Autodesk Fusion 360 part; units mm, degrees
sketch "Bottom back base" plane through (0, 0, 0) normal (0, 0, 1) x (1, 0, 0)
  line L0 (-60, 60) -> (-60, -60)
  line L1 (60, -20) -> (60, 20)
  line L2 (-60, 0) -> (-57.5, 0) construction
  line L3 (-57.5, -60) -> (-57.5, -6) construction
  line L4 (-57.5, -6) -> (12.5, -6) construction
  line L5 (12.5, -6) -> (12.5, -34) construction
  line L6 (12.5, -34) -> (30, -34)
  line L7 (30, -34) -> (12.5, -34)
  line L8 (12.5, -34) -> (-40, -34)
  line L9 (-40, -34) -> (-40, -60)
  line L10 (30, -34) -> (30, -60)
  line L11 (-40, 34) -> (-40, 60)
  line L12 (12.5, 34) -> (-40, 34)
  line L13 (12.5, 34) -> (30, 34)
  line L14 (30, 34) -> (30, 60)
  line L15 (50, -60) -> (60, -20)
  line L16 (50, 60) -> (60, 20)
  line L17 (50, 60) -> (30, 60)
  line L18 (-40, 60) -> (-60, 60)
  line L19 (-60, -60) -> (-40, -60)
  line L20 (30, -60) -> (50, -60)
  point P0 (60, 60)
  point P1 (60, -60)
  dimension "d1" = 120
  dimension "d2" = 120
  dimension "d3" = 2.5
  dimension "d4" = 54
  dimension "d5" = 70
  dimension "d6" = 28
  dimension "d8" = 70
  dimension "d9" = 10
  dimension "d10" = 40
  dimension "d11" = 10
  dimension "d12" = 40
extrude "Bottom back height" add sketch "Bottom back base" along normal blind 5
sketch "Connector" plane through (-60, 0, 0) normal (-1, 0, 0) x (0, -1, 0)
  line L0 (-60, 0) -> (60, 0)
  line L1 (60, 0) -> (60, 5)
  line L2 (60, 5) -> (-60, 5)
  line L3 (-60, 5) -> (-60, 0)
  line L4 (0, 0) -> (0, 5) construction
  line L5 (30, 4) -> (-30, 4)
  line L6 (-30, 4) -> (-30, 1)
  line L7 (-30, 1) -> (30, 1)
  line L8 (30, 1) -> (30, 4)
  line L9 (30, 4) -> (-30, 1) construction
  line L10 (-30, 4) -> (30, 1) construction
  point P0 (0, 2.5)
  dimension "d15" = 3
  dimension "d16" = 60
extrude "Connector width" add sketch "Connector" along normal blind 60 contours L5 L6 L7 L8
equation "d6 = 54 mm - 26 mm"
Geometry: final body of the model. Coordinates: model frame, mm. A direction names the side the tool comes from. Round coordinates to 2 decimals unless told otherwise and drop trailing zeros. Order: outer loops, then holes, each group sorted by start corner. A loop starts at its lowest first (then second) coordinate and runs counter-clockwise, first axis right, second up. Notation, with made-up numbers: M 23.25,-6.5 L 47.25,-6.5 A31 cw 47.25,17.5 Z; hole C 42,64 d3. An arc over 180 degrees is marked long. Use one line per item in the form item = value. Start each with the question number.
Q1. Pin query (flat end, axial travel): pin 1 Ø2.5 at (y, z) = (42.5, 3.5) entering from +X; pin 2 Ø2 at (x, z) = (-96.5, 1.5) entering from -Y; pin 3 Ø2.5 at (y, z) = (-49, 3.5) entering from +X. Return the tip coordinate at first contact, or that it passes through.
Q2. Cut plane D-D (x = -8). Return loops of the section in (y, z), and give its area (3 significant figures).
Q3. Mould query, pull axis X, two halves, no side actions, for faces 1 (the face through (-40, 47, 2)), 2 (the face through (-5, 34, 2)), 3 (the face through (60, 0, 2)), 4 (the face through (-90, 0, 4)). Classes: +X half, -X half, draft (parallel to the pull), parting line (faces both ways), or undercut.
Q4. Cut plane B-B (y = -10). Return loops of the section in (x, z), and give its area (3 significant figures).
Q5. Cut plane C-C (z = 2). Return loops of the section in (x, y).
Q6. Access query for faces 5 (the face through (-90, 0, 1)), 6 (the face through (-40, -47, 2)), 7 (the face through (30, 47, 2)). Directions: +Z, -Z, +X, -X, +Y, -Y. A direction counts if a zero-diameter tool reaches every point of the face in a straight line with its end or side. Return the directions, or none.
Q7. Cut plane A-A (y = -38.5). Return loops of the section in (x, z) (3 decimals).
Q8. Material intervals for line 1 (Y direction, x = -83.5, z = 2.75); line 2 (Z direction, x = -69.5, y = 2); line 3 (X direction, y = 47.5, z = 2.8) (3 decimals), sorted ascending. Write a range as [from, to].
Geometry results:
q1.pin_1 = 54.69
q1.pin_2 = -30
q1.pin_3 = 53.06
q2.outline = M -34,0 L 34,0 L 34,5 L -34,5 Z
q2.area = 340 mm^2
q3.face_1 = undercut
q3.face_2 = undercut
q3.face_3 = +X half
q3.face_4 = draft
q4.outline = M -120,1 L -60,1 L -60,0 L 60,0 L 60,5 L -60,5 L -60,4 L -120,4 Z
q4.area = 780 mm^2
q5.outline = M -120,-30 L -60,-30 L -60,-60 L -40,-60 L -40,-34 L 30,-34 L 30,-60 L 50,-60 L 60,-20 L 60,20 L 50,60 L 30,60 L 30,34 L -40,34 L -40,60 L -60,60 L -60,30 L -120,30 Z
q6.face_5 = -Z, -X, +Y, -Y
q6.face_6 = +Z, -Z, -Y
q6.face_7 = +Z, -Z, +Y
q7.outline = M -60,0 L -40,0 L -40,5 L -60,5 Z; M 30,0 L 55.375,0 L 55.375,5 L 30,5 Z
q8.line_1 = [-30, 30]
q8.line_2 = [1, 4]
q8.line_3 = [-60, -40], [30, 53.125]
